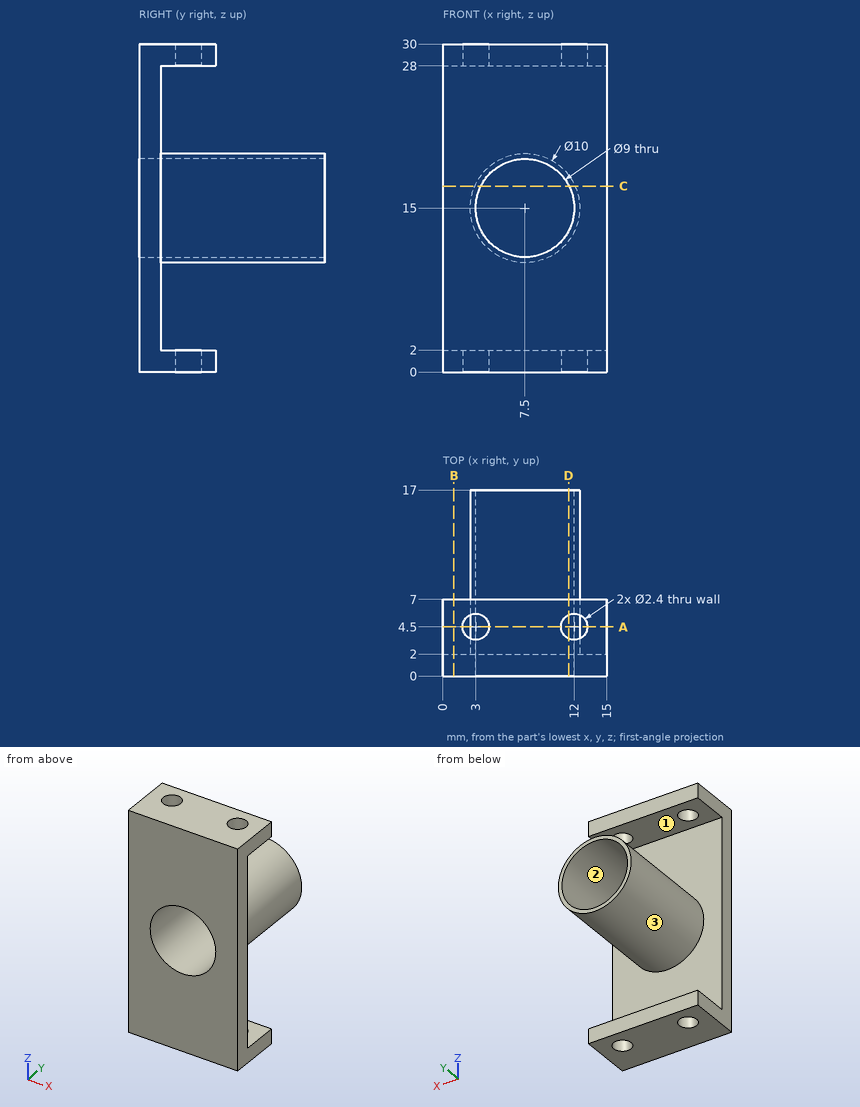
Geometry check sheet. Reference: drawing and pictorial views, mm from the part's lowest x, y, z. Give positions to 0.01 mm unless a question says otherwise; leave off trailing zeros. Write each loop counter-clockwise with the first axis right and the second up, starting at its lowest first coordinate (ties: lowest second). Pieces come first, ordered by that corner, then holes. Notation, with made-up numbers: (-27.5, -34) -> (15.5, -34) arc R19 ccw to (15.5, -28) -> close; hole circle Ø8 at (6, 4.25). An arc over 180 degrees is marked (long way). One line per item, written item: value. Start each with the question number.
Item 1: Section check C-C on z = 17. Record the cut outline in (x, y), then the cut area to 3 significant figures.
Item 2: Section check D-D on x = 11.5. Record the cut outline in (y, z).
Item 3: Section check B-B on x = 1. Record the cut outline in (y, z).
Item 4: Section check A-A on y = 4.5. Record the cut outline in (x, z).
Item 5: Draft check along X on the marked faces 1, 2 and 3. Enter one of: +X half, -X half, draft (parallel to the pull), parting line (faces both ways), or undercut.
Item 6: Material ranges on probe 1 along Y at (x, z) = (12, 29.15); probe 2 along Z at (x, y) = (6, 4.25); probe 3 along Z at (x, y) = (14.5, 5), recorded low to high. Write a range as from..to.
Item 7: Gauge pin test, flat ends, axial feed: pin 1 (8 mm diameter, centred on y = 8, z = 7.5, fed in from -X); pin 2 (2 mm diameter, centred on y = 11.5, z = 12.5, fed in from +X); pin 3 (1.9 mm diameter, centred on x = 12, y = 4.5, fed in from -Z). Record the tip position at first contact, or that the pin passes through.
Results list:
1. outline: (0, 0) -> (3.47, 0) -> (3.47, 17) -> (2.92, 17) -> (2.92, 2) -> (0, 2) -> close; (11.53, 0) -> (15, 0) -> (15, 2) -> (12.08, 2) -> (12.08, 17) -> (11.53, 17) -> close
1. area: 30.4 mm²
2. outline: (0, 0) -> (3.41, 0) -> (3.41, 2) -> (2, 2) -> (2, 12) -> (17, 12) -> (17, 12.94) -> (0, 12.94) -> close; (0, 17.06) -> (17, 17.06) -> (17, 18) -> (2, 18) -> (2, 28) -> (3.41, 28) -> (3.41, 30) -> (0, 30) -> close; (5.59, 0) -> (7, 0) -> (7, 2) -> (5.59, 2) -> close; (5.59, 28) -> (7, 28) -> (7, 30) -> (5.59, 30) -> close
3. outline: (0, 0) -> (7, 0) -> (7, 2) -> (2, 2) -> (2, 28) -> (7, 28) -> (7, 30) -> (0, 30) -> close
4. outline: (0, 0) -> (1.8, 0) -> (1.8, 2) -> (0, 2) -> close; (0, 28) -> (1.8, 28) -> (1.8, 30) -> (0, 30) -> close; circle Ø10 at (7.5, 15); (4.2, 0) -> (10.8, 0) -> (10.8, 2) -> (4.2, 2) -> close; (4.2, 28) -> (10.8, 28) -> (10.8, 30) -> (4.2, 30) -> close; (13.2, 0) -> (15, 0) -> (15, 2) -> (13.2, 2) -> close; (13.2, 28) -> (15, 28) -> (15, 30) -> (13.2, 30) -> close; hole circle Ø9 at (7.5, 15)
5. face 1: draft
5. face 2: undercut
5. face 3: parting line
6. probe 1: 0..3.3, 5.7..7
6. probe 2: 0..2, 10.23..10.76, 19.24..19.77, 28..30
6. probe 3: 0..2, 28..30
7. pin 1: x = 3.93
7. pin 2: x = 12.27
7. pin 3: z = 11.48
